from build123d import *

# Parameters (mm, degrees)
CYLINDER_R               = 20
CYLINDER_DEPTH           = 100
CYLINDER_PLACEMENT_ANGLE = 295
PAD_DEPTH                = 120
POCKET_DEPTH             = 80.001
SKETCH003_R              = 12
PAD001_DEPTH             = 15
SKETCH004_R              = 8
POCKET001_DEPTH          = 65.001


with BuildPart() as cilindro:
    # Cylinder → Cylinder (new body)
    with BuildSketch(Plane.XY):
        Circle(CYLINDER_R)
    extrude(amount=CYLINDER_DEPTH)


with BuildPart() as cilindro_1:
    # Cylinder placement: moved
    add(cilindro.part.moved(Location((0, -45.315389, -1.130913))).rotate(Axis((0, -45.315389, -1.130913), (1, 0, 0)), CYLINDER_PLACEMENT_ANGLE))


with BuildPart() as cut:
    # Sketch → Pad (new body)
    with BuildSketch(Plane.XZ):
        with BuildLine():
            Line((-33, 20), (33, 20))
            ThreePointArc((40, 13), (37.949747, 17.949747), (33, 20))
            Line((40, 13), (40, 0))
            Line((40, 0), (-40, 0))
            Line((-40, 0), (-40, 13))
            ThreePointArc((-33, 20), (-37.949747, 17.949747), (-40, 13))
        make_face()
    extrude(amount=-PAD_DEPTH)

    # Sketch002 → Pocket (cut, through all)
    with BuildSketch(Plane(origin=(40, 0, 0), x_dir=(0, 0, 1), z_dir=(1, 0, 0))):
        with BuildLine():
            Line((0, -80), (6.738911, -80))
            ThreePointArc((12.738911, -86), (10.981552, -81.757359), (6.738911, -80))
            Line((12.738911, -86), (12.738911, -134.292511))
            Line((12.738911, -134.292511), (0, -134.292511))
            Line((0, -134.292511), (0, -80))
        make_face()
    extrude(amount=-POCKET_DEPTH, mode=Mode.SUBTRACT)

    # Sketch003 → Pad001 (new body)
    with BuildSketch(Plane.XZ):
        with BuildLine():
            Line((-40, 0), (40, 0))
            Line((40, 0), (21.770267, -32.290463))
            ThreePointArc((-21.770267, -32.290463), (0, -45), (21.770267, -32.290463))
            Line((-40, 0), (-21.770267, -32.290463))
        make_face()
        with Locations((0, -20)):
            Circle(SKETCH003_R, mode=Mode.SUBTRACT)
    extrude(amount=-PAD001_DEPTH)

    # Sketch004 → Pocket001 (cut, through all)
    with BuildSketch(Plane(origin=(0, 0, 20), x_dir=(-1, 0, 0), z_dir=(0, 0, 1))):
        with Locations((17, -100)):
            Circle(SKETCH004_R)
        with Locations((-17, -100)):
            Circle(SKETCH004_R)
        with Locations((-17, -60)):
            Circle(SKETCH004_R)
        with Locations((17, -60)):
            Circle(SKETCH004_R)
    extrude(amount=-POCKET001_DEPTH, mode=Mode.SUBTRACT)

    # Cut: cut Cilindro
    add(cilindro_1.part, mode=Mode.SUBTRACT)


solid = cut.part
Model file for the job. Use its own axes, mm. A direction names the side the tool comes from. Give positions to 0.01 mm unless a question says otherwise; leave off trailing zeros. Order: outer loops, then holes, each group sorted by start corner. A loop starts at its lowest first (then second) coordinate and runs counter-clockwise, first axis right, second up. Notation, with made-up numbers: M -11.5,54.5 L 38.5,54.5 A14 ccw 38.5,62.5 Z; hole C -17,65 d3. An arc over 180 degrees is marked long. Put each result on its own line as item: value. Start each with the question number.
(1) Pull direction X, two halves, no side cores. Call faces 3 (the face through (0, 7, -45)), 4 (the face through (0, 72, 20)), 5 (the face through (0.44, 18.28, 6.46)), 6 (the face through (-40, 32, 6)): released by +X, released by -X, zero draft, split by the parting line, or undercut.
(2) Band-saw the part on B-B on x = 0. Give the cut face in (y, z).
(3) Pin check, flat tips, straight feed: pin 1 Ø12 at (x, z) = (-21, 12.5) entering from -Y; pin 2 Ø5 at (x, y) = (-31, 46.5) entering from -Z; pin 3 Ø10 at (x, y) = (-14, 104) entering from -Z; pin 4 Ø1.5 at (y, z) = (15, -33.5) entering from +X. Stop position of each tip, or through.
(4) Band-saw the part on A-A on y = 100. Give the cut face in (x, z), then the cut area to 3 significant figures.
(5) Tool access for faces 1 (the face through (1, 47, 0)), 2 (the face through (-15.959, 52.068, 10.14)): list every direction of +Z, -Z, +X, -X, +Y, -Y with a clear straight run to the whole face (end or side of a thin tool).
(6) Band-saw the part on C-C on x = -23.5. Give the cut face in (y, z), then the cut area to 3 significant figures.
(7) Drill centre lines: L1, parallel to X at y = 60, z = 4.5; L2, parallel to Y at x = -17, z = 5.25; L3, parallel to X at y = 100, z = 17. Where is each one in solid material? Low to high. Write a range as [from, to].
(8) Band-saw the part on D-D on z = -20. Give the cut face in (x, y), then the cut area to 3 significant figures.
Results below:
1. face 3: split by the parting line
1. face 4: zero draft
1. face 5: undercut
1. face 6: released by -X
2. outline: M 0,-45 L 15,-45 L 15,-32 L 0,-32 Z; M 0,-8 L 15,-8 L 15,0 L 80,0 L 80,6.74 A6 cw 86,12.74 L 120,12.74 L 120,20 L 47.32,20 L 0,-2.07 Z
3. pin 1: stops at y = 0
3. pin 2: stops at z = 0
3. pin 3: stops at z = 12.74
3. pin 4: stops at x = 21.5
4. outline: M -40,12.74 L -25,12.74 L -25,20 L -33,20 A7 ccw -40,13 Z; M -9,12.74 L 9,12.74 L 9,20 L -9,20 Z; M 25,12.74 L 40,12.74 L 40,13 A7 ccw 33,20 L 25,20 Z
4. area: 328 mm2
5. face 1: -Z, +X, -X, +Y
5. face 2: +Z, -Z
6. outline: M 0,-29.23 L 15,-29.23 L 15,0 L 55.34,0 L 55.34,20 L 0,20 Z; M 64.66,0 L 80,0 L 80,6.74 A6 cw 86,12.74 L 95.34,12.74 L 95.34,20 L 64.66,20 Z; M 104.66,12.74 L 120,12.74 L 120,20 L 104.66,20 Z
6. area: 2,080 mm2
7. L1: x = [-40, -25], [-9, 9], [25, 40]
7. L2: y = [0, 52], [68, 80]
7. L3: x = [-38.74, -25], [-9, 9], [25, 38.74]
8. outline: M -28.71,0 L -12,0 L -12,15 L -28.71,15 Z; M 12,0 L 28.71,0 L 28.71,15 L 12,15 Z
8. area: 501 mm2
